Part print with two shaded views. Sizes in mm from the minimum x, y, z corner. Round coordinates to 2 decimals unless told otherwise and drop trailing zeros. Loops run counter-clockwise (first coordinate to the right, second up) from the corner with the lowest first, then second, coordinate; pieces in that order, holes last.
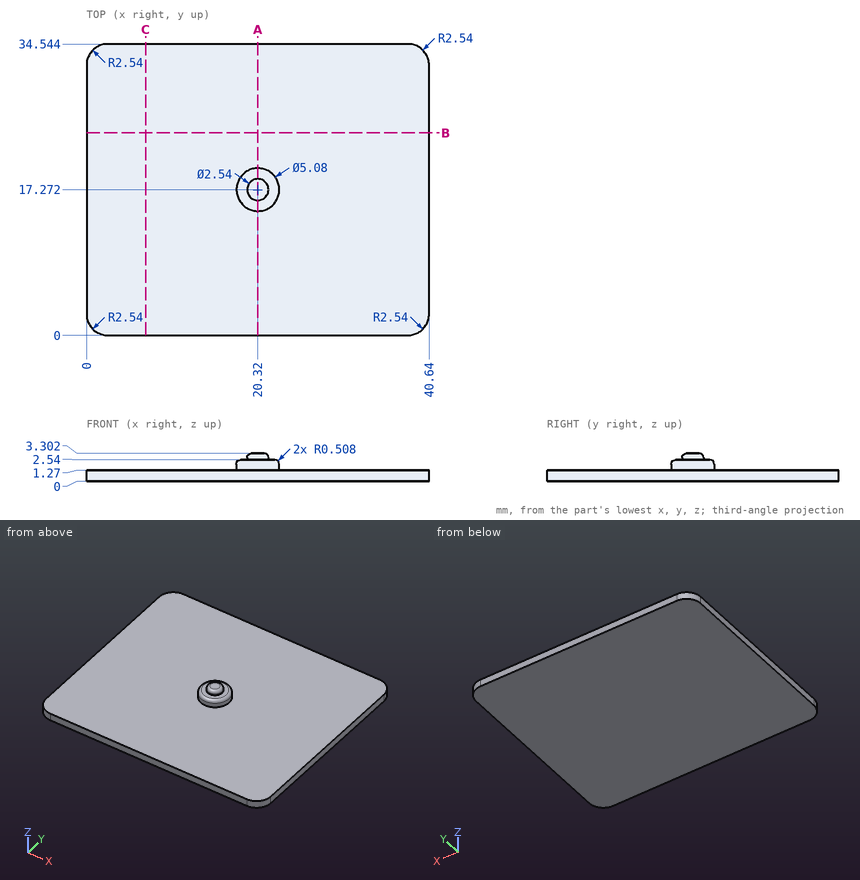
Item 1: Cut at A-A (x = 20.32). List the corners of the cut face in (y, z), plus the area to 3 significant figures.
Verdict:
outline: (0, 0) - (34.54, 0) - (34.54, 1.27) - (19.81, 1.27) - (19.81, 2.03) arc R0.51 ccw to (19.3, 2.54) - (18.54, 2.54) - (18.54, 2.79) arc R0.51 ccw to (18.03, 3.3) - (16.51, 3.3) arc R0.51 ccw to (16, 2.79) - (16, 2.54) - (15.24, 2.54) arc R0.51 ccw to (14.73, 2.03) - (14.73, 1.27) - (0, 1.27) - close
area: 52.0 mm2
Item 2: Wall check: L1, parallel to Z at x = 12, y = 12; L2, parallel to Y at x = 20.5, z = 1.45; L3, parallel to Y at x = 21, z = 2.6. Give the ranges that are in metal, low to high.
Verdict:
L1: z = 0 to 1.27
L2: y = 14.74 to 19.81
L3: y = 16.2 to 18.34
Item 3: Flat gauge pin, fed straight in: P1, Ø4, axis at x = 12.5, y = 24.5, coming from the +Z side. Where does the tip first touch, or does it go through?
Verdict:
P1: stops at z = 1.27
Item 4: Cut at B-B (y = 24). List the corners of the cut face in (x, z), plus the area to 3 significant figures.
Verdict:
outline: (0, 0) - (40.64, 0) - (40.64, 1.27) - (0, 1.27) - close
area: 51.6 mm2
Item 5: Cut at C-C (x = 7). List the corners of the cut face in (y, z).
Verdict:
outline: (0, 0) - (34.54, 0) - (34.54, 1.27) - (0, 1.27) - close
